For this review, take the finished solid that the model builds, in its own axes (mm). Round coordinates to 2 decimals unless told otherwise and drop trailing zeros. Loops run counter-clockwise (first coordinate to the right, second up) from the corner with the lowest first, then second, coordinate; pieces in that order, holes last.
1) Wall thickness on L1, parallel to Y at x = -24.15, z = 12.7; L2, parallel to Z at x = -13.5, y = 253 (3 decimals); L3, parallel to X at y = 119, z = 21.75 (3 decimals): over which ranges is each line inside the solid? List them lowest first.
2) Take a section at B-B (x = -9.5). State the section outline as (y, z) points (1 decimal), then the cut area to 3 significant figures.
3) Take a section at A-A (y = 397). State the section outline as (x, z) points (3 decimals).
4) Insertion check: pin 1 (8 mm diameter, centred on y = 12.7, z = 12.7, fed in from +X). The pin has a flat end and moves straight along its axis. Give the tip position at first contact, or say it passes through.
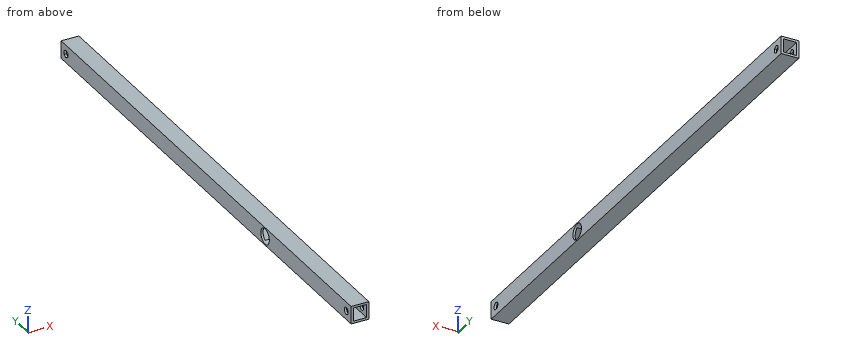
Autodesk Inventor part; units mm, degrees
ref_plane "YZ Plane" through (0, 0, 0) normal (1, 0, 0) x (0, 1, 0)
ref_plane "XZ Plane" through (0, 0, 0) normal (0, 1, 0) x (-1, 0, 0)
ref_plane "XY Plane" through (0, 0, 0) normal (0, 0, 1) x (1, 0, 0)
sketch "Sketch1" plane through (0, 0, 0) normal (0, 1, 0) x (-1, 0, 0)
  line L0 (0, 0) -> (25.4, 0)
  line L1 (25.4, 0) -> (25.4, 25.4)
  line L2 (25.4, 25.4) -> (0, 25.4)
  line L3 (0, 25.4) -> (0, 0)
  line L4 (3.175, 3.175) -> (22.225, 3.175)
  line L5 (22.225, 3.175) -> (22.225, 22.225)
  line L6 (22.225, 22.225) -> (3.175, 22.225)
  line L7 (3.175, 22.225) -> (3.175, 3.175)
  dimension "d0" = 25.4
  dimension "d1" = 25.4
  dimension "d2" = 3.175
  dimension "d3" = 3.175
  dimension "d4" = 3.175
  dimension "d6" = 3.175
extrude "Extrusion1" add sketch "Sketch1" along normal blind 762
sketch "Sketch3" plane through (0, 0, 25.4) normal (1, 0, 0) x (0, 0, -1)
  circle A0 centre (12.7, 12.7) radius 5.08
  line L0 (25.4, 0) -> (25.4, 762)
  line L1 (0, 0) -> (25.4, 0)
  dimension "d17" = 10.16
  dimension "d18" = 12.7
  dimension "d19" = 12.7
extrude "Extrusion3" cut sketch "Sketch3" against normal blind 25.4
sketch "Sketch4" plane through (0, 0, 25.4) normal (1, 0, 0) x (0, 0, -1)
  line L0 (0, 0) -> (0, 762)
  line L1 (0, 0) -> (25.4, 0)
  line L2 (25.4, 0) -> (25.4, 762)
  point P0 (12.7, 12.7)
  dimension "d22" = 12.7
  dimension "d23" = 12.7
sketch "Sketch5" plane through (0, 0, 25.4) normal (1, 0, 0) x (0, 0, -1)
  line L0 (15.4496, 744.5375) -> (9.9504, 744.5375)
  line L1 (9.9504, 744.5375) -> (7.2007, 749.3)
  line L2 (7.2007, 749.3) -> (9.9504, 754.0625)
  line L3 (9.9504, 754.0625) -> (15.4496, 754.0625)
  line L4 (15.4496, 754.0625) -> (18.1993, 749.3)
  line L5 (18.1993, 749.3) -> (15.4496, 744.5375)
  line L6 (0, 0) -> (0, 762)
  line L7 (0, 762) -> (25.4, 762)
  point P0 (25.4, 0)
  point P1 (12.7, 749.3)
  point P2 (12.7, 744.5375)
  dimension "d29" = 9.525
  dimension "d30" = 12.7
  dimension "d31" = 12.7
extrude "Extrusion5" cut sketch "Sketch5" against normal blind 25.4
extrude "Extrusion7" [suppressed]
sketch "Sketch6" plane through (0, 0, 25.4) normal (1, 0, 0) x (0, 0, -1)
  circle A0 centre (12.7, 226.06) radius 11.1125
  line L0 (25.4, 0) -> (25.4, 762)
  line L1 (0, 0) -> (25.4, 0)
  dimension "d40" = 22.225
  dimension "d41" = 12.7
  dimension "d42" = 226.06
extrude "Extrusion8" cut sketch "Sketch6" against normal blind 25.4
equation "\"d4\" = d2"
properties part number "1x1 8th Inch Aluminum Tube Custom Lift Arms"
Response:
1. L1: y = 0 to 7.62, 17.78 to 214.95, 237.17 to 744.54, 754.06 to 762
1. L2: z = 0 to 3.175, 22.225 to 25.4
1. L3: x = -25.4 to -22.225, -3.175 to 0
2. outline: (0, 0) - (762, 0) - (762, 3.2) - (231.8, 3.2) arc R11.1 cw to (220.3, 3.2) - (0, 3.2) - close; (0, 22.2) - (220.3, 22.2) arc R11.1 cw to (231.8, 22.2) - (762, 22.2) - (762, 25.4) - (0, 25.4) - close
2. area: 4,810 mm2
3. outline: (-25.4, 0) - (0, 0) - (0, 25.4) - (-25.4, 25.4) - close; hole (-22.225, 3.175) - (-3.175, 3.175) - (-3.175, 22.225) - (-22.225, 22.225) - close
4. pin 1: passes through
